```python
from build123d import *

# Parameters (mm, degrees)
SKETCH2_R           = 137.922
SKETCH2_R_2         = 122.682
BOSS_EXTRUDE2_DEPTH = 1.5875
SKETCH3_W           = 290.977734258
SKETCH3_H           = 504.828840158
CUT_EXTRUDE1_DEPTH  = 138.922
CUT_EXTRUDE2_DEPTH  = 4.175


with BuildPart() as part:
    # Sketch2 → Boss-Extrude2 (new body, symmetric)
    with BuildSketch(Plane(origin=(248.273568551, -245.01347209, 0), x_dir=(0, -1, 0), z_dir=(0, 0, -1))):
        with Locations((-257.71347209, 248.273568551)):
            Circle(SKETCH2_R)
        with Locations((-257.71347209, 248.273568551)):
            Circle(SKETCH2_R_2, mode=Mode.SUBTRACT)
    extrude(amount=BOSS_EXTRUDE2_DEPTH, both=True)

    # Sketch3 → Cut-Extrude1 (cut, through all)
    with BuildSketch(Plane(origin=(0, 0, 0), x_dir=(0, 0, -1), z_dir=(1, 0, 0))):
        with Locations((4.206907001, 10.947122083)):
            Rectangle(SKETCH3_W, SKETCH3_H)
    extrude(amount=CUT_EXTRUDE1_DEPTH, mode=Mode.SUBTRACT)

    # Sketch5 → Cut-Extrude2 (cut, through all)
    with BuildSketch(Plane.XY.offset(1.5875)):
        with BuildLine():
            Line((-3.302, 150.582467631), (-3.302, 141.732))
            Line((-3.302, 141.732), (0, 141.732))
            Line((0, 141.732), (0, 150.622))
            ThreePointArc((0, 150.622), (-1.651118319, 150.612116554), (-3.302, 150.582467631))
        make_face()
        with BuildLine():
            Line((-109.043255392, 81.788598611), (-116.699944513, 86.209190137))
            ThreePointArc((-116.699944513, 86.209190137), (-117.591747875, 84.773982239), (-118.465901574, 83.327956562))
            Line((-118.465901574, 83.327956562), (-110.732355392, 78.862991592))
            Line((-110.732355392, 78.862991592), (-109.043255392, 81.788598611))
        make_face()
        with BuildLine():
            Line((-114.354109205, -47.189929975), (-122.010798327, -51.610521501))
            ThreePointArc((-122.010798327, -51.610521501), (-121.213773508, -53.100449816), (-120.398555388, -54.580501964))
            Line((-120.398555388, -54.580501964), (-112.665009205, -50.115536994))
            Line((-112.665009205, -50.115536994), (-114.354109205, -47.189929975))
        make_face()
        with BuildLine():
            Line((-3.302, -116.332), (-3.302, -125.182467631))
            ThreePointArc((-3.302, -125.182467631), (-1.651118319, -125.212116554), (0, -125.222))
            Line((0, -125.222), (0, -116.332))
            Line((0, -116.332), (-3.302, -116.332))
        make_face()
    extrude(amount=-CUT_EXTRUDE2_DEPTH, mode=Mode.SUBTRACT)


solid = part.part
```
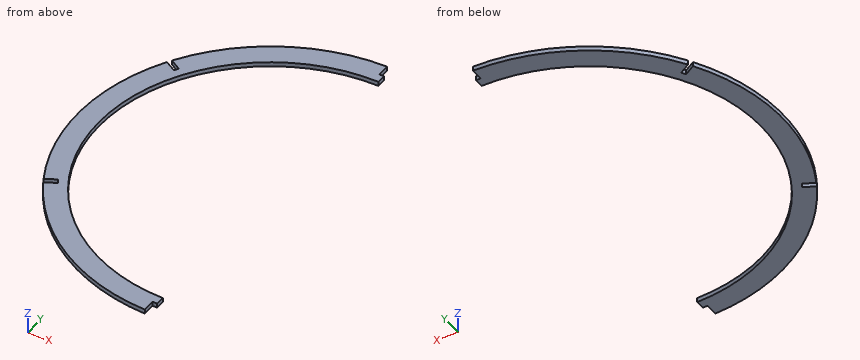
Can you work these out from the model? Positions are in its coordinate system, mm. Coordinates: 2 decimals unless noted, no trailing zeros. Write each loop counter-clockwise with the first axis right and the second up, starting at its lowest first coordinate (ties: lowest second). Pieces come first, ordered by that corner, then holes. Notation, with made-up numbers: M 72,35.5 L 99,35.5 A15 cw 99,40.5 Z; hole C -20.75,10.5 d1. An arc over 180 degrees is marked long. Write item = value, one per line. Start each with the question number.
Q1. If I drill on L1, parallel to Y at x = -77, z = 0.4; L2, parallel to Y at x = -79.5, z = 1.5; L3, parallel to X at y = 79, z = 0.65, over which ranges is the centre line in solid material (lowest first)? Write a range as [from, to].
Q2. If we section it at A-A, the plane x = -41: Write out the boundary of the cut face in (y, z).
Q3. If we section it at C-C, the plane x = -104: Write out the boundary of the cut face in (y, z), then the cut area to 3 significant figures.
Q4. If we section it at D-D, the plane y = -18: Write out the boundary of the cut face in (x, z).
Q5. I'm going to push flat-ended pins straight in: pin 1 (1.6 mm diameter, centred on x = -1.5, z = 0, fed in from -Y); pin 2 (1.5 mm diameter, centred on x = -33.5, z = 0, fed in from -Y); pin 3 (1.6 mm diameter, centred on y = -121, z = -0.5, fed in from +X); pin 4 (12 mm diameter, centred on x = -39, y = -93.5, fed in from -Z). Where does each tip first touch, or does it pass through?
Q6. If we section it at B-B, the plane z = -0.6: Write out the boundary of the cut face in (x, y) (1 decimal), then the cut area to 3 significant figures.
Check sheet entries:
q1.L1 = [-101.73, -82.81], [108.21, 127.13]
q1.L2 = [-100, -80.74], [106.14, 125.4]
q1.L3 = [-120.94, -110.97], [-110.65, -103.22]
q2.outline = M -118.99,-1.59 L -102.93,-1.59 L -102.93,1.59 L -118.99,1.59 Z; M 128.33,-1.59 L 144.39,-1.59 L 144.39,1.59 L 128.33,1.59 Z
q3.outline = M -77.89,-1.59 L -52.38,-1.59 L -52.38,1.59 L -77.89,1.59 Z; M 77.78,-1.59 L 103.29,-1.59 L 103.29,1.59 L 77.78,1.59 Z
q3.area = 162 mm²
q4.outline = M -134.46,-1.59 L -118.78,-1.59 L -118.78,1.59 L -134.46,1.59 Z
q5.pin_1 = -116.33
q5.pin_2 = -121.28
q5.pin_3 = -3.3
q5.pin_4 = through
q6.outline = M -122,-51.6 L -114.4,-47.2 L -112.7,-50.1 L -120.4,-54.6 A137.9 ccw -3.3,-125.2 L -3.3,-116.3 L 0,-116.3 L 0,-110 A122.7 cw 0,135.4 L 0,141.7 L -3.3,141.7 L -3.3,150.6 A137.9 ccw -116.7,86.2 L -109,81.8 L -110.7,78.9 L -118.5,83.3 A137.9 ccw Z
q6.area = 6,120 mm²
